Verification items for the finished model (mm, model axes). Give positions to 0.01 mm unless a question says otherwise; leave off trailing zeros. Loops run counter-clockwise (first coordinate to the right, second up) from the corner with the lowest first, then second, coordinate; pieces in that order, holes last. Notation, with made-up numbers: (54.25, -20.5) -> (103.25, -20.5) arc R24 ccw to (103.25, -8.5) -> close; hole circle Ø8 at (47.5, -21.5). An arc over 180 degrees is marked (long way). Use one line per item in the form item = value. Start each with the question number.
from build123d import *

# Parameters (mm, degrees)
SKETCH_1_W          = 30
SKETCH_1_H          = 40
SKETCH_1_W_2        = 26
SKETCH_1_H_2        = 36
EXTRUDE_1_DEPTH     = 444
SKETCH_2_R          = 4
CUT_EXTRUDE_1_DEPTH = 96


with BuildPart() as part:
    # 草图1 → 凸台-拉伸1 (new body)
    with BuildSketch(Plane.XY):
        with Locations((-3.063208411, -0.691053078)):
            Rectangle(SKETCH_1_W, SKETCH_1_H)
        with Locations((-3.063208411, -0.691053078)):
            Rectangle(SKETCH_1_W_2, SKETCH_1_H_2, mode=Mode.SUBTRACT)
    extrude(amount=EXTRUDE_1_DEPTH)

    # 草图2 → 切除-拉伸1 (cut)
    with BuildSketch(Plane.ZY.offset(18.063208411)):
        with Locations((396, -0.691053078)):
            Circle(SKETCH_2_R)
        with Locations((428, -0.691053078)):
            Circle(SKETCH_2_R)
        with Locations((16, -0.691053078)):
            Circle(SKETCH_2_R)
        with Locations((48, -0.691053078)):
            Circle(SKETCH_2_R)
        with Locations((93, -0.691053078)):
            Circle(SKETCH_2_R)
        with Locations((351, -0.691053078)):
            Circle(SKETCH_2_R)
    extrude(amount=-CUT_EXTRUDE_1_DEPTH, mode=Mode.SUBTRACT)


solid = part.part
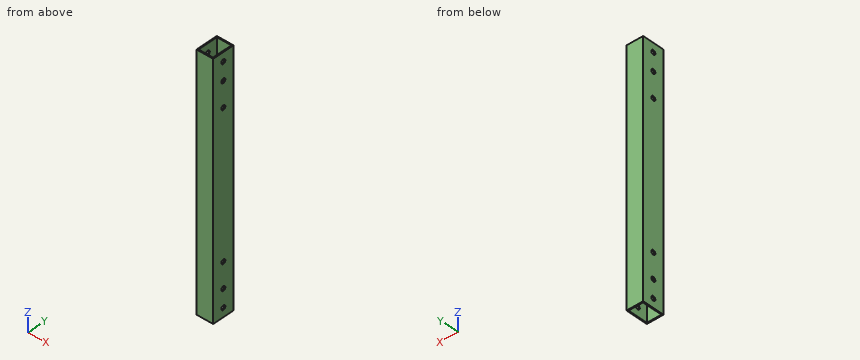
Item 1: Sectioned sample at C-C, the plane z = 428. Enter the section's corners in (x, y).
Item 2: Sectioned sample at A-A, the plane x = -8.75. Enter the section's corners in (y, z), and give its area (3 significant figures).
Item 3: Gauge pin test, flat end, axial feed: pin 1 Ø9 at (y, z) = (-0.69, 396) entering from +X. Record the tip position at first contact, or that the pin passes through.
Item 4: Material ranges on line 1 (X direction, y = -8, z = 193); line 2 (Y direction, x = -3, z = 66); line 3 (Y direction, x = -17.4, z = 428), recorded low to high.
Item 5: Sectioned sample at B-B, the plane y = 9. Enter the section's corners in (x, z).
Outcome:
q1.outline = (-18.06, -20.69) -> (11.94, -20.69) -> (11.94, -4.69) -> (9.94, -4.69) -> (9.94, -18.69) -> (-16.06, -18.69) -> (-16.06, -4.69) -> (-18.06, -4.69) -> close; (-18.06, 3.31) -> (-16.06, 3.31) -> (-16.06, 17.31) -> (9.94, 17.31) -> (9.94, 3.31) -> (11.94, 3.31) -> (11.94, 19.31) -> (-18.06, 19.31) -> close
q2.outline = (-20.69, 0) -> (-18.69, 0) -> (-18.69, 444) -> (-20.69, 444) -> close; (17.31, 0) -> (19.31, 0) -> (19.31, 444) -> (17.31, 444) -> close
q2.area = 1,780 mm^2
q3.pin_1 = 11.94
q4.line_1 = -18.06 to -16.06, 9.94 to 11.94
q4.line_2 = -20.69 to -18.69, 17.31 to 19.31
q4.line_3 = -20.69 to -4.69, 3.31 to 19.31
q5.outline = (-18.06, 0) -> (-16.06, 0) -> (-16.06, 444) -> (-18.06, 444) -> close; (9.94, 0) -> (11.94, 0) -> (11.94, 444) -> (9.94, 444) -> close
